Autodesk Inventor part; units mm, degrees
ref_plane "YZ Plane" through (0, 0, 0) normal (1, 0, 0) x (0, 1, 0)
ref_plane "XZ Plane" through (0, 0, 0) normal (0, 1, 0) x (-1, 0, 0)
ref_plane "XY Plane" through (0, 0, 0) normal (0, 0, 1) x (1, 0, 0)
sketch "Sketch1" plane through (0, 0, 0) normal (0, 0, 1) x (1, 0, 0)
  line L0 (-9.7234, 29.9641) -> (9.7234, 29.9641)
  line L1 (9.7234, 29.9641) -> (9.7234, -29.9641)
  line L2 (9.7234, -29.9641) -> (-9.7234, -29.9641)
  line L3 (-9.7234, -29.9641) -> (-9.7234, 29.9641)
  point P0 (0, 0)
  point P1 (9.7234, 0)
  point P2 (0, -29.9641)
  dimension "d0" = 19.4469
  dimension "d1" = 59.9281
extrude "Extrusion1" add sketch "Sketch1" along normal blind 1.5875
sketch "Sketch2" plane through (0, 0, 1.5875) normal (0, 0, 1) x (1, 0, 0)
  line L0 (-9.7234, -29.9641) -> (9.7234, -29.9641)
  line L1 (9.7234, -29.9641) -> (9.7234, 14.8828)
  line L2 (9.7234, -29.9641) -> (9.7234, 29.9641)
  line L3 (-9.7234, 29.9641) -> (-9.7234, -29.9641)
  line L4 (-9.7234, -29.9641) -> (-9.7234, 14.8828)
  line L5 (-9.7234, 14.8828) -> (-0.7937, 23.8125)
  line L6 (-9.7234, 14.8828) -> (2.905, 14.8828) construction
  line L7 (9.7234, 14.8828) -> (4.7625, 19.8437)
  line L8 (9.7234, 14.8828) -> (16.7393, 14.8828) construction
  line L9 (6.9453, 22.8203) -> (6.9453, 17.6609)
  line L10 (-6.9453, 22.8203) -> (-6.9453, 17.6609)
  line L11 (-6.9453, 22.8203) -> (-9.7234, 25.5984)
  line L12 (6.9453, 22.8203) -> (9.7234, 25.5984)
  line L13 (-9.7234, 25.5984) -> (-9.7234, 14.8828)
  line L14 (9.7234, 25.5984) -> (9.7234, 14.8828)
  point P0 (0, 0)
  dimension "d4" = 44.8469
  dimension "d5" = 44.8469
  dimension "d6" = 45
  dimension "d7" = 135
  dimension "d8" = 5.1594
  dimension "d9" = 5.1594
  dimension "d10" = 2.7781
  dimension "d11" = 2.7781
  dimension "d12" = 0
  dimension "d13" = 0
extrude "Extrusion2" cut sketch "Sketch2" against normal blind 1.5875
sketch "Sketch3" plane through (0, 0, 1.5875) normal (0, 0, 1) x (1, 0, 0)
  line L0 (9.7234, 29.9641) -> (-9.7234, 29.9641)
  line L1 (-3.6711, 29.9641) -> (3.6711, 29.9641)
  line L2 (3.6711, 29.9641) -> (3.6711, 27.3844)
  line L3 (3.6711, 27.3844) -> (-3.6711, 27.3844)
  line L4 (-3.6711, 27.3844) -> (-3.6711, 29.9641)
  point P0 (0, 0)
  point P1 (0, 27.3844)
  dimension "d16" = 7.3422
  dimension "d17" = 2.5797
extrude "Extrusion3" add sketch "Sketch3" along normal blind 3.9688
sketch "Sketch4" plane through (-9.7234, 29.9641, 0) normal (0, 1, 0) x (1, 0, 0)
  circle A0 centre (12.6008, -5.1594) radius 0.3969
  circle A1 centre (9.7226, -5.1594) radius 0.3969
  circle A2 centre (6.8461, -5.1594) radius 0.3969
  line L0 (13.3945, -1.5875) -> (13.3945, -5.5563)
  line L1 (13.3945, -5.5563) -> (6.0523, -5.5563)
  line L2 (6.0523, -1.5875) -> (6.0523, -5.5563)
  point P0 (9.7234, 0)
  dimension "d20" = 0.7937
  dimension "d21" = 0.7937
  dimension "d22" = 0.7937
  dimension "d23" = 0.7937
  dimension "d24" = 0.3969
  dimension "d25" = 0.7937
  dimension "d26" = 0.3969
  dimension "d27" = 0.3969
  dimension "d28" = 7.3422
  dimension "d29" = 3.6703
extrude "Extrusion4" add sketch "Sketch4" along normal blind 6.35
properties part number "Water Sensor"
The model under review builds one solid part; all positions refer to its coordinate system, in mm. A direction names the side the tool comes from. Give positions to 0.01 mm unless a question says otherwise; leave off trailing zeros. Order: outer loops, then holes, each group sorted by start corner. A loop starts at its lowest first (then second) coordinate and runs counter-clockwise, first axis right, second up. Notation, with made-up numbers: M 71,81.25 L 129,81.25 A29 cw 129,118.25 Z; hole C 58.25,83 d7. An arc over 180 degrees is marked long. One line per question, with ' | ' between items. Start each with the question number.
1) Consider section C-C, the plane y = -9. Give the boundary of the cut face in (x, z), then the cut area to 3 significant figures.
2) Clearance check with flat-ended pins moving along their axes: P1, Ø1, axis at x = 5.5, z = 1.5, coming from the +Y side; P2, Ø3, axis at y = 28.5, z = 4, coming from the +X side; P3, Ø9.5, axis at x = 2, y = 7, coming from the +Z side. State where each tip first meets the part, or that it passes through.
3) Wall thickness on L1, parallel to Y at x = 3.5, z = 5.05; L2, parallel to Y at x = 5.25, z = 0.75; L3, parallel to Z at x = 6.25, y = 4: over which ranges is each line inside the solid? List them lowest first. Write a range as from..to.
4) Consider section D-D, the plane z = 2.2. Give the boundary of the cut face in (x, y).
5) For faces 1 (the face through (-8.354, 16.252, 0.805)), 2 (the face through (6.945, 20, 1)), 3 (the face through (3.671, 29, 4)), 4 (the face through (0, 27.384, 4)), 5 (the face through (-3.671, 29, 4)), list the 3-axis set-ups (+Z, -Z, +X, -X, +Y, -Y) from which the entire face can be reached by the end or side of a thin tool; tool diameter is ignored.
6) Consider section B-B, the plane x = -1.75. Give the boundary of the cut face in (y, z), then the cut area to 3 significant figures.
7) Consider section A-A, the plane x = 7.5. Give the boundary of the cut face in (y, z) (1 decimal).
Found:
1) outline: M -9.72,0 L 9.72,0 L 9.72,1.59 L -9.72,1.59 Z | area: 30.9 mm²
2) P1: stops at y = 29.96 | P2: stops at x = 3.67 | P3: stops at z = 1.59
3) L1: y = 27.38..29.96 | L2: y = -29.96..29.96 | L3: z = 0..1.59
4) outline: M -3.67,27.38 L 3.67,27.38 L 3.67,29.96 L -3.67,29.96 Z
5) face 1: +Z, -Z, -X | face 2: +Z, -Z, +X | face 3: +Z, +X, +Y, -Y | face 4: +Z, +X, -X, -Y | face 5: +Z, -X, +Y, -Y
6) outline: M -29.96,0 L 29.96,0 L 29.96,5.56 L 27.38,5.56 L 27.38,1.59 L -29.96,1.59 Z | area: 105 mm²
7) outline: M -30,0 L 17.1,0 L 17.1,1.6 L -30,1.6 Z; M 23.4,0 L 30,0 L 30,1.6 L 23.4,1.6 Z
